from build123d import *

# Parameters (mm, degrees)
F0_R      = 14.637001
F1_DEPTH  = 68.58
F2_SIZE   = 5.08
F1_FACE_R = 9.557001
F3_DEPTH  = 16.764


with BuildPart() as f1:
    # F0 (on Top) → F1 (new body)
    with BuildSketch(Plane.XY):
        with Locations((-54.797947, 12.446093)):
            Circle(F0_R)
    extrude(amount=F1_DEPTH)

    # F2
    f2_edges = [f1.edges().sort_by_distance(p)[0] for p in [
        (-69.434948, 12.446093, 68.58),
    ]]
    chamfer(f2_edges, length=F2_SIZE)

    # F1_face (on face) → F3 (join)
    with BuildSketch(Plane(origin=(-54.797947, 12.446093, 68.58), x_dir=(1, 0, 0), z_dir=(0, 0, 1))):
        Circle(F1_FACE_R)
    extrude(amount=F3_DEPTH)


solid = f1.part
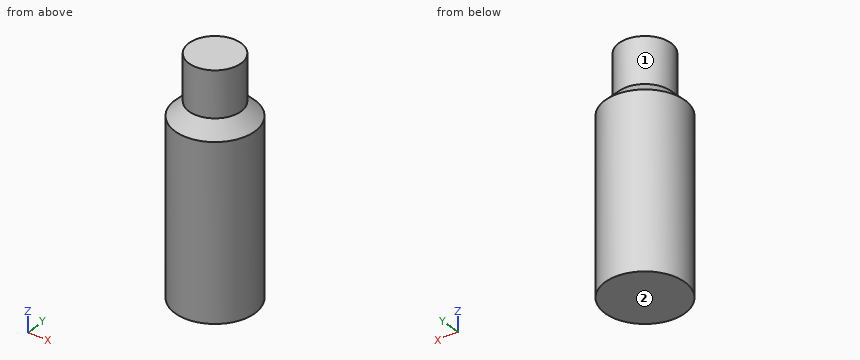
Can you work these out from the model? Positions are in its coordinate system, mm. Face numbers are marked on the shaded views. A direction names the side the tool comes from. Coordinates: 2 decimals unless noted, no trailing zeros. Write each loop counter-clockwise with the first axis right and the second up, starting at its lowest first coordinate (ties: lowest second). Pieces come first, ordered by that corner, then holes. Notation, with made-up numbers: (43, 41.5) - (61, 41.5) arc R18 cw to (61, 46.5) - close; hole circle Ø6 at (-19.5, 36.25). An arc over 180 degrees is marked (long way). Return JSON: item names as keys, results as strings. Group by question number.
Item 1: If we section it at A-A (z = 65): Write out the boundary of the cut face in (x, y), then the cut area to 3 significant figures.
Item 2: I'm going to push flat-ended pins straight in: pin 1 Ø8 at (y, z) = (22, 46.5) entering from +X; pin 2 Ø12 at (y, z) = (23.5, 68) entering from +X; pin 3 Ø5 at (x, z) = (-45.5, 63) entering from +Y. Where does each tip first touch, or does it pass through?
Item 3: Please list where these lines run through material, in increasing order: probe 1 along Z at (x, y) = (-49, 0.75); probe 2 along X at (y, z) = (1.75, 32); probe 3 along Y at (x, z) = (-63.5, 34).
Item 4: If we section it at B-B (z = 54): Write out the boundary of the cut face in (x, y).
Item 5: Which directions (+Z, -Z, +X, -X, +Y, -Y) give clear straight access to the entire face, cutting with the end or side of a thin tool? Please do the marked faces 1 and 2.
Return value:
{
 "1": {"outline": "circle Ø26.27 at (-54.8, 12.45)", "area": "542 mm^2"},
 "2": {"pin 1": "stops at x = -41.26", "pin 2": "stops at x = -41.99", "pin 3": "stops at y = 25.41"},
 "3": {"probe 1": "z = 0 to 65.08", "probe 2": "x = -64.79 to -44.81", "probe 3": "y = 0.68 to 24.22"},
 "4": {"outline": "circle Ø29.27 at (-54.8, 12.45)"},
 "5": {"face 1": "+Z", "face 2": "-Z, +X, -X, +Y, -Y"}
}
